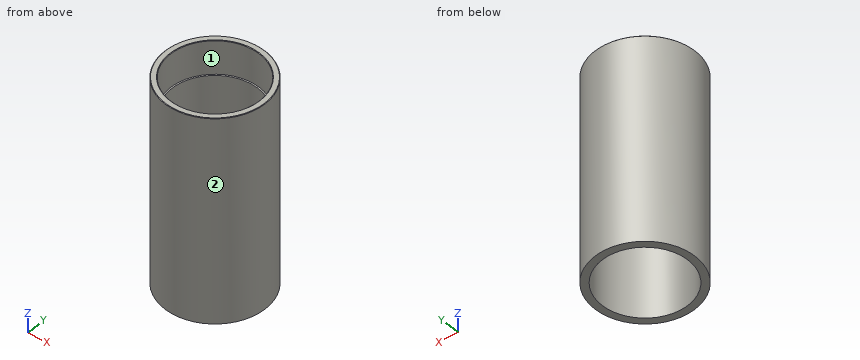
from build123d import *

# Parameters (mm, degrees)
F0_R     = 24.5
F0_R_2   = 21
F1_DEPTH = 100
F2_R     = 21.725
F2_R_2   = 21
F3_DEPTH = 16.5
F4_SIZE  = 0.25


with BuildPart() as f1:
    # F0 (on Top) → F1 (new body)
    with BuildSketch(Plane.XY):
        Circle(F0_R)
        Circle(F0_R_2, mode=Mode.SUBTRACT)
    extrude(amount=F1_DEPTH)

    # F2 (on face) → F3 (cut)
    with BuildSketch(Plane.XY.offset(100)):
        Circle(F2_R)
        Circle(F2_R_2, mode=Mode.SUBTRACT)
    extrude(amount=-F3_DEPTH, mode=Mode.SUBTRACT)

    # F4
    f4_edges = [f1.edges().sort_by_distance(p)[0] for p in [
        (-24.5, 0, 100),
        (-21.725, 0, 100),
    ]]
    chamfer(f4_edges, length=F4_SIZE)


solid = f1.part
Build history of the part. All positions in model axes, mm. Face numbers are marked on the shaded views. Round coordinates to 2 decimals unless told otherwise and drop trailing zeros. Loops run counter-clockwise (first coordinate to the right, second up) from the corner with the lowest first, then second, coordinate; pieces in that order, holes last. Notation, with made-up numbers: (-8.75, 20) -> (6.25, 20) arc R14 cw to (6.25, 29) -> close; hole circle Ø10 at (31.25, 44). An arc over 180 degrees is marked (long way). Answer in a Markdown table with one row per item.
Item 1: Pin check, flat tips, straight feed: pin 1 (1 mm diameter, centred on x = 1, z = 52, fed in from +Y); pin 2 (4 mm diameter, centred on x = 7.5, z = 57, fed in from +Y); pin 3 (1.5 mm diameter, centred on x = -18.5, z = 23.5, fed in from -Y). Stop position of each tip, or through.
Answers below:
| item | result |
|---|---|
| pin 1 | stops at y = 24.49 |
| pin 2 | stops at y = 23.87 |
| pin 3 | stops at y = -16.89 |
Item 2: Saw through at A-A (x = 0). Write the cut outline in (y, z) (3 decimals).
Answers below:
| item | result |
|---|---|
| outline | (-24.5, 0) -> (-21, 0) -> (-21, 83.5) -> (-21.725, 83.5) -> (-21.725, 99.75) -> (-21.975, 100) -> (-24.25, 100) -> (-24.5, 99.75) -> close; (21, 0) -> (24.5, 0) -> (24.5, 99.75) -> (24.25, 100) -> (21.975, 100) -> (21.725, 99.75) -> (21.725, 83.5) -> (21, 83.5) -> close |
Item 3: Saw through at D-D (z = 92.5). Write the cut outline in (x, y) (3 decimals).
Answers below:
| item | result |
|---|---|
| outline | circle Ø49 at (0, 0); hole circle Ø43.45 at (0, 0) |
Item 4: Saw through at C-C (z = 58.5). Write the cut outline in (x, y).
Answers below:
| item | result |
|---|---|
| outline | circle Ø49 at (0, 0); hole circle Ø42 at (0, 0) |
Item 5: Mould opens along Y. For the marked faces 1 and 2 say: +Y half, -Y half, draft (parallel to the pull), parting line (faces both ways), or undercut.
Answers below:
| item | result |
|---|---|
| face 1 | undercut |
| face 2 | parting line |
Item 6: Drill centre lines: L1, parallel to Y at x = 0, z = 65; L2, parallel to Y at x = 0, z = 92 (3 decimals); L3, parallel to X at y = 14.5, z = 42.5. Where is each one in solid material? Low to high. Write a range as [from, to].
Answers below:
| item | result |
|---|---|
| L1 | y = [-24.5, -21], [21, 24.5] |
| L2 | y = [-24.5, -21.725], [21.725, 24.5] |
| L3 | x = [-19.75, -15.19], [15.19, 19.75] |
